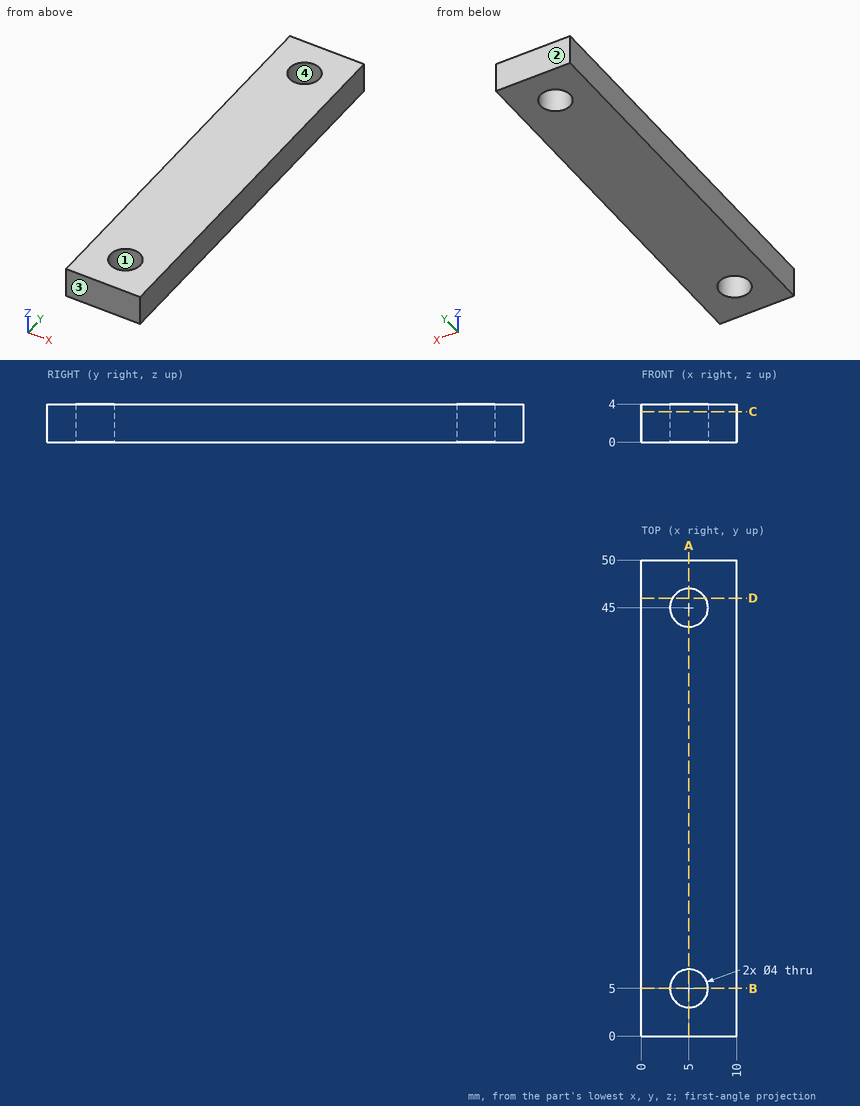
Design review of the part shown in the three views and the two pictorial views. Dimensions are in mm from the part's minimum x, y and z. Give positions to 0.01 mm unless a question says otherwise; leave off trailing zeros. Write each loop counter-clockwise with the first axis right and the second up, starting at its lowest first coordinate (ties: lowest second). Pieces come first, ordered by that corner, then holes. Notation, with made-up numbers: M -4.5,80 L 50.5,80 A17 cw 50.5,104 Z; hole C 11,8.25 d4. An arc over 180 degrees is marked long. Answer as CSV lines item,"result".
1. Consider section C-C, the plane z = 3.2. Write out the cut boundary in (x, y).
Findings:
outline,"M 0,0 L 10,0 L 10,50 L 0,50 Z; hole C 5,5 d4; hole C 5,45 d4"
2. Draft analysis for pull direction Y (two halves, no side actions). For the marked faces 1, 2, 3 and 4, state which applies: +Y half, -Y half, draft (parallel to the pull), parting line (faces both ways), or undercut.
Findings:
face 1,"undercut"
face 2,"+Y half"
face 3,"-Y half"
face 4,"undercut"
3. Wall thickness on line 1 (Y direction, x = 5, z = 2.6); line 2 (Y direction, x = 3.5, z = 0.6); line 3 (X direction, y = 6, z = 0.9): over which ranges is each line inside the solid? List them lowest first.
Findings:
line 1,"y = 0 to 3, 7 to 43, 47 to 50"
line 2,"y = 0 to 3.68, 6.32 to 43.68, 46.32 to 50"
line 3,"x = 0 to 3.27, 6.73 to 10"
4. For pin 1 (2 mm diameter, centred on y = 42.5, z = 1.5, fed in from -X); pin 2 (3 mm diameter, centred on x = 5, y = 5, fed in from -Z), all flat-tipped, find the tip position at first contact; note any pin that passes through.
Findings:
pin 1,"stops at x = 0"
pin 2,"passes through"
5. Consider section A-A, the plane x = 5. Write out the cut boundary in (y, z).
Findings:
outline,"M 0,0 L 3,0 L 3,4 L 0,4 Z; M 7,0 L 43,0 L 43,4 L 7,4 Z; M 47,0 L 50,0 L 50,4 L 47,4 Z"
6. Consider section D-D, the plane y = 46. Write out the cut boundary in (x, z).
Findings:
outline,"M 0,0 L 3.27,0 L 3.27,4 L 0,4 Z; M 6.73,0 L 10,0 L 10,4 L 6.73,4 Z"
7. Consider section B-B, the plane y = 5. Write out the cut boundary in (x, z).
Findings:
outline,"M 0,0 L 3,0 L 3,4 L 0,4 Z; M 7,0 L 10,0 L 10,4 L 7,4 Z"
